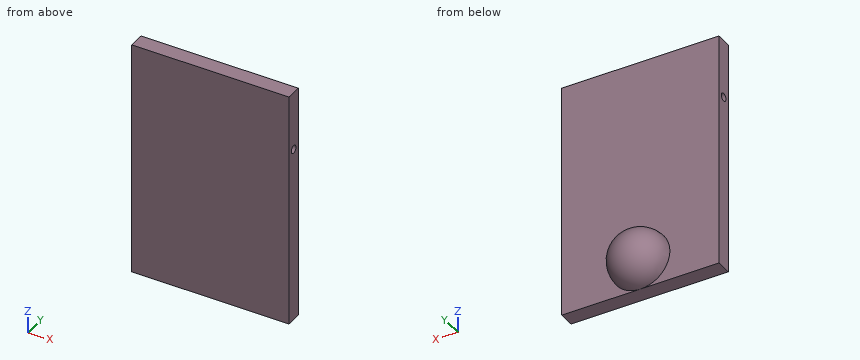
```python
from build123d import *

# Parameters (mm, degrees)
SKETCH_1_W          = 100
SKETCH_1_H          = 150
EXTRUDE_1_DEPTH     = 10
REVOLVE_2_ANGLE     = 180
SKETCH_3_R          = 2.5
CUT_EXTRUDE_1_DEPTH = 129.263644498


with BuildPart() as part:
    # 草圖1 → 填料-伸長1 (new body)
    with BuildSketch(Plane(origin=(0, 0, 0), x_dir=(1, 0, 0), z_dir=(0, 1, 0))):
        Rectangle(SKETCH_1_W, SKETCH_1_H)
    extrude(amount=EXTRUDE_1_DEPTH)

    # 草圖2 → 旋轉2 (revolve)
    with BuildSketch(Plane(origin=(0, 10, 0), x_dir=(1, 0, 0), z_dir=(0, 1, 0))):
        with BuildLine():
            Line((0, 75), (0, 37.5))
            ThreePointArc((0, 37.5), (18.75, 56.25), (0, 75))
        make_face()
    revolve(axis=Axis((0, 10, -75), (0, 0, 1)), revolution_arc=REVOLVE_2_ANGLE)

    # 草圖3 → 除料-伸長1 (cut, through all)
    with BuildSketch(Plane.ZY.offset(50)):
        with Locations((37.5, 5)):
            Circle(SKETCH_3_R)
    extrude(amount=-CUT_EXTRUDE_1_DEPTH, mode=Mode.SUBTRACT)


solid = part.part
```
CAD build for the part. Positions are in the model's coordinates, mm. Coordinates: 2 decimals unless noted, no trailing zeros. Order: outer loops, then holes, each group sorted by start corner. A loop starts at its lowest first (then second) coordinate and runs counter-clockwise, first axis right, second up. Notation, with made-up numbers: (63.25, 52.5) - (68.25, 52.5) arc R27 cw to (68.25, 91.5) - close; hole circle Ø3 at (86.5, 2.25). An arc over 180 degrees is marked (long way). Use a Markdown table: item, result. Add a question column.
(1) Flat gauge pins, fed straight in: pin 1 (12 mm diameter, centred on y = 18.5, z = 35.5, fed in from +X); pin 2 (12 mm diameter, centred on x = 39.5, z = 26, fed in from +Y). Where does each tip first touch, or does it go through?
(2) Saw through at B-B (y = 5). Give the cut face in (x, z), then the cut area to 3 significant figures.
(3) Drill centre lines: line 1 along Y through (x, z) = (16, 37.5); line 2 along Y through (x, z) = (14, 37); line 3 along Y through (x, z) = (25.5, -21). Where is each one in solid material? Low to high. Write a range as [from, to].
(4) Saw through at D-D (z = -48). Give the cut face in (x, y), then the cut area to 3 significant figures.
(5) Saw through at C-C (x = 36). Give the cut face in (y, z), then the cut area to 3 significant figures.
(6) Saw through at A-A (z = 37.5). Give the cut face in (x, y), then the cut area to 3 significant figures.
Solved:
| question | item | result |
|---|---|---|
| 1 | pin 1 | passes through |
| 1 | pin 2 | stops at y = 10 |
| 2 | outline | (-50, -75) - (50, -75) - (50, 35) - (-50, 35) - close; (-50, 40) - (50, 40) - (50, 75) - (-50, 75) - close |
| 2 | area | 14,500 mm² |
| 3 | line 1 | y = [0, 2.5], [7.5, 10] |
| 3 | line 2 | y = [0, 2.55], [7.45, 10] |
| 3 | line 3 | y = [0, 10] |
| 4 | outline | (-50, 0) - (50, 0) - (50, 10) - (16.84, 10) arc R16.84 ccw to (-16.84, 10) - (-50, 10) - close |
| 4 | area | 1,450 mm² |
| 5 | outline | (0, -75) - (10, -75) - (10, 75) - (0, 75) - close; hole circle Ø5 at (5, 37.5) |
| 5 | area | 1,480 mm² |
| 6 | outline | (-50, 0) - (50, 0) - (50, 2.5) - (-50, 2.5) - close; (-50, 7.5) - (50, 7.5) - (50, 10) - (-50, 10) - close |
| 6 | area | 500 mm² |
